Source: CAD feature listing. Evaluate the final solid. Frame: model axes, mm. Face numbers are marked on the shaded views. A direction names the side the tool comes from. Round coordinates to 2 decimals unless told otherwise and drop trailing zeros. Loops run counter-clockwise (first coordinate to the right, second up) from the corner with the lowest first, then second, coordinate; pieces in that order, holes last. Notation, with made-up numbers: (71, 0.25) - (106, 0.25) arc R13 cw to (106, 22.25) - close; hole circle Ø8 at (-3, 89.5). An arc over 180 degrees is marked (long way). One line per question, with ' | ' between items.
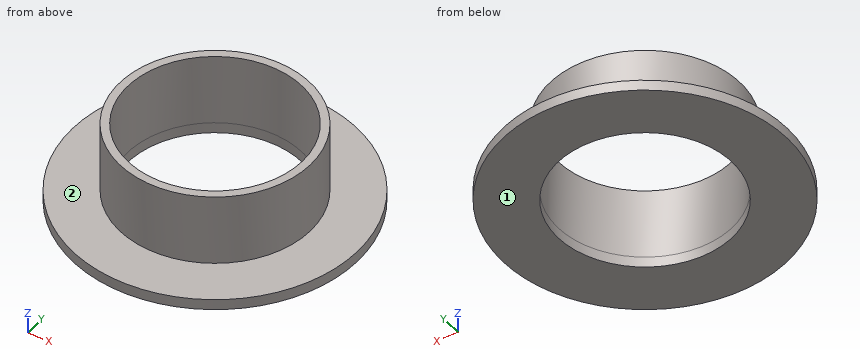
from build123d import *

# Parameters (mm, degrees)
F0_R     = 40
F1_DEPTH = 3
F2_R     = 26.75
F2_R_2   = 24.5
F3_DEPTH = 20
F4_DEPTH = 3.001


with BuildPart() as f1:
    # F0 (on Top) → F1 (new body)
    with BuildSketch(Plane.XY):
        Circle(F0_R)
    extrude(amount=F1_DEPTH)

    # F2 (on face) → F3 (join)
    with BuildSketch(Plane.XY.offset(3)):
        Circle(F2_R)
        Circle(F2_R_2, mode=Mode.SUBTRACT)
    extrude(amount=F3_DEPTH)

    # F2 (on face) → F4 (cut, through all)
    with BuildSketch(Plane.XY.offset(3)):
        Circle(F2_R_2)
    extrude(amount=-F4_DEPTH, mode=Mode.SUBTRACT)


solid = f1.part
1. Contact query for flat-ended pins moving along their axis: P1, Ø1, axis at y = -25, z = 17, coming from the +X side; P2, Ø6, axis at x = 24.5, z = 3.5, coming from the -Y side; P3, Ø3, axis at x = -17, z = 7, coming from the -Y side. Output: stop coordinate, or through.
Worked out:
P1: stops at x = 10.74 | P2: stops at y = -33.7 | P3: stops at y = -21.8
2. Access query for the marked faces 1 and 2. Directions: +Z, -Z, +X, -X, +Y, -Y. A direction counts if a zero-diameter tool reaches every point of the face in a straight line with its end or side. Return the directions, or none.
Worked out:
face 1: -Z, +X, -X, +Y, -Y | face 2: +Z
3. Section query C-C, the plane z = 19. Return loops of the section in (x, y), plus the area to 3 significant figures.
Worked out:
outline: circle Ø53.5 at (0, 0); hole circle Ø49 at (0, 0) | area: 362 mm2
4. Section query D-D, the plane x = 28.5. Return loops of the section in (y, z), plus the area to 3 significant figures.
Worked out:
outline: (-28.07, 0) - (28.07, 0) - (28.07, 3) - (-28.07, 3) - close | area: 168 mm2
5. Material intervals for probe 1 along Z at (x, y) = (26, -23); probe 2 along X at (y, z) = (22.5, 10.25); probe 3 along X at (y, z) = (-15.5, 15.5), sorted ascending.
Worked out:
probe 1: z = 0 to 3 | probe 2: x = -14.47 to -9.7, 9.7 to 14.47 | probe 3: x = -21.8 to -18.97, 18.97 to 21.8
6. Section query A-A, the plane y = 0. Return loops of the section in (x, z), plus the area to 3 significant figures.
Worked out:
outline: (-40, 0) - (-24.5, 0) - (-24.5, 23) - (-26.75, 23) - (-26.75, 3) - (-40, 3) - close; (24.5, 0) - (40, 0) - (40, 3) - (26.75, 3) - (26.75, 23) - (24.5, 23) - close | area: 183 mm2
